Geometry: see drawing. Coordinates: mm, zero at the bounding-box minimum. Coordinates: 2 decimals unless noted, no trailing zeros. Loops run counter-clockwise (first coordinate to the right, second up) from the corner with the lowest first, then second, coordinate; pieces in that order, holes last.
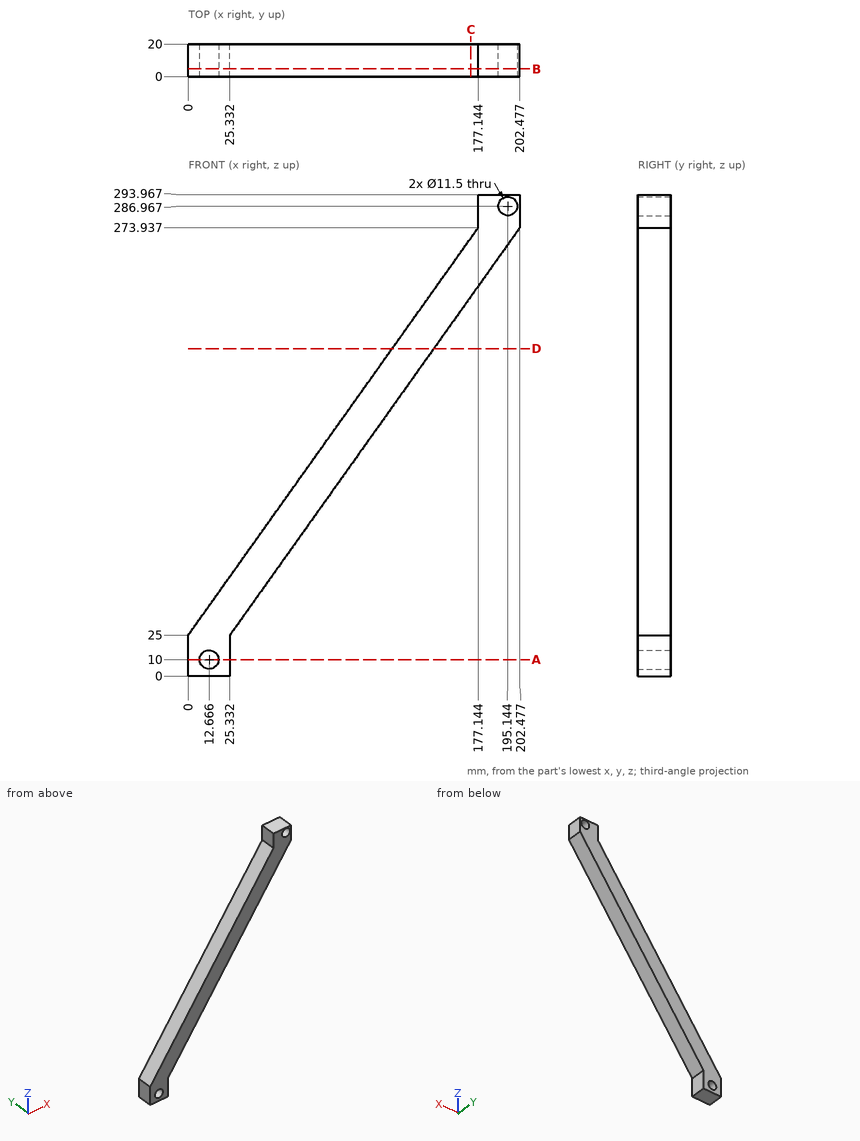
Item 1: Section query B-B (y = 4.75). Count the separate pieces of the cut face and the enclosed holes in it, then the cut area to 3 significant figures.
Result:
separate pieces: 1
enclosed holes: 2
area: 7,240 mm2
Item 2: Section query D-D (z = 200). Output: boundary loops of the cut face in (x, y), then the cut area to 3 significant figures.
Result:
outline: (124.53, 0) - (149.86, 0) - (149.86, 20) - (124.53, 20) - close
area: 507 mm2
Item 3: Section query A-A (z = 10). Output: boundary loops of the cut face in (x, y), then the cut area to 3 significant figures.
Result:
outline: (0, 0) - (6.92, 0) - (6.92, 20) - (0, 20) - close; (18.42, 0) - (25.33, 0) - (25.33, 20) - (18.42, 20) - close
area: 277 mm2
Item 4: Section query C-C (x = 172.5). Output: boundary loops of the cut face in (y, z).
Result:
outline: (0, 231.81) - (20, 231.81) - (20, 267.41) - (0, 267.41) - close
Item 5: Contact query for flat-ended pins moving along their axis: P1, Ø1.5, axis at x = 110, y = 6.5, coming from the +Z side (1 decimal); P2, Ø6, axis at y = 17.5, z = 95, coming from the -X side; P3, Ø2, axis at y = 8, z = 122, coming from the -X side (1 decimal). Output: stop coordinate, or through.
Result:
P1: stops at z = 180.6
P2: stops at x = 47.68
P3: stops at x = 68.3
Item 6: Line query: L1, parallel to X at y = 11.75, z = 10; L2, parallel to Z at x = 15.5, y = 6.75 (1 decimal); L3, parallel to Z at x = 143.5, y = 10.25 (1 decimal). Output: solid intervals per line, ascending.
Result:
L1: x = 0 to 6.92, 18.42 to 25.33
L2: z = 0 to 5, 15 to 46.8
L3: z = 191.1 to 226.7
